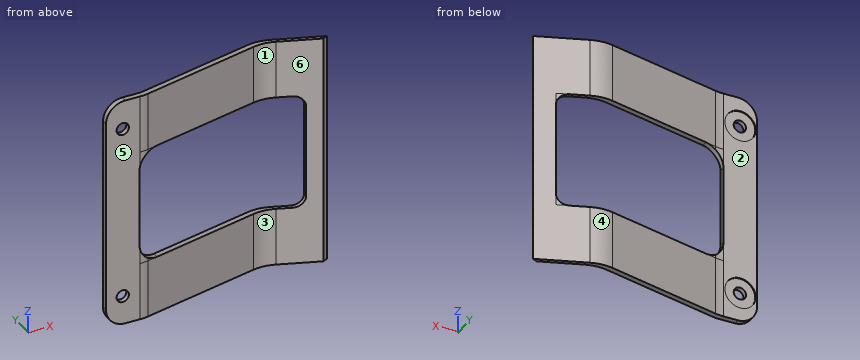
from build123d import *

# Parameters (mm, degrees)
EXTRUDE_1_DEPTH                 = 60
FILLET_1_R                      = 10
CHAMFER_1_SIZE                  = 2
CHAMFER_1_SIZE_2                = 1.558687347
CUT_EXTRUDE_1_REACH             = 86.761
SKETCH_2_R                      = 1.6
SKETCH_3_R                      = 4
CUT_EXTRUDE_2_DEPTH             = 0.2
CUT_EXTRUDE_3_REACH             = 86.761
SKETCH_4_W                      = 45.702932162
SKETCH_4_H                      = 30
CUT_EXTRUDE_3_DIRECTION_2_REACH = 86.761
FILLET_2_OUTLINE_W              = 8.702446171
FILLET_2_OUTLINE_H              = 1.5
FILLET_2_DEPTH                  = 5
FILLET_START                    = 55
FILLET_2_2_OUTLINE_W            = 8.702446171
FILLET_2_2_OUTLINE_H            = 1.5
FILLET_2_2_DEPTH                = 5
FILLET_2_3_DEPTH                = 1.3
FILLET_START_2                  = 1.3
FILLET_2_4_DEPTH                = 0.2
FILLET_START_3                  = 1.478876
FILLET_2_5_DEPTH                = 0.906082345
FILLET_START_4                  = 15
FILLET_2_6_DEPTH                = 30
FILLET_3_R                      = 3


with BuildPart() as part:
    # 草图1 → 凸台-拉伸1 (new body)
    with BuildSketch(Plane.XY):
        Polygon((0, 0), (10, 0), (45, 8), (60, 2.5), (60, 3.565103021), (44.204382552, 9.356829418), (9.830753848, 1.5), (0, 1.5), align=None)
    extrude(amount=EXTRUDE_1_DEPTH)

    # 圆角1
    fillet_1_edges = [part.edges().sort_by_distance(p)[0] for p in [
        (9.830753848, 1.5, 30),
        (44.204382552, 9.356829418, 30),
        (45, 8, 30),
        (10, 0, 30),
    ]]
    fillet(fillet_1_edges, radius=FILLET_1_R)

    # 倒角1
    # the kernel refuses this chamfer: 2, 1.558687347 mm, written as the material it takes off along each edge
    with BuildSketch(Plane(origin=(60, 2.5, -5.143365976), x_dir=(-0.9388763158866087, 0.3442546491584233, 0), z_dir=(0, 0, 1))) as chamfer_1_piece_1:
        Polygon((CHAMFER_1_SIZE, 0), (CHAMFER_1_SIZE_2 * 0.3442546492, -CHAMFER_1_SIZE_2 * 0.938876315999), (0, 0), align=None)
    extrude(amount=70.286731952, mode=Mode.SUBTRACT)

    # 草图2 → 切除-拉伸1 (cut, up to next)
    with BuildSketch(Plane(origin=(0, 1.5, 0), x_dir=(1, 0, 0), z_dir=(0, 1, 0)), mode=Mode.PRIVATE) as cut_extrude_1_sk1:
        with Locations(Location((4.351223085, -7.5, 0), (0, 0, 270))):
            Circle(SKETCH_2_R)
    cut_extrude_1_tool1 = extrude(cut_extrude_1_sk1.sketch, amount=-CUT_EXTRUDE_1_REACH, mode=Mode.PRIVATE) & part.part
    # 草图2 → 切除-拉伸1 (cut, up to next)
    with BuildSketch(Plane(origin=(0, 1.5, 0), x_dir=(1, 0, 0), z_dir=(0, 1, 0)), mode=Mode.PRIVATE) as cut_extrude_1_sk2:
        with Locations(Location((4.351223085, -52.5, 0), (0, 0, 270))):
            Circle(SKETCH_2_R)
    cut_extrude_1_tool2 = extrude(cut_extrude_1_sk2.sketch, amount=-CUT_EXTRUDE_1_REACH, mode=Mode.PRIVATE) & part.part
    add(cut_extrude_1_tool1.solids().sort_by_distance((4.351223, 1.5, 7.5))[0], mode=Mode.SUBTRACT)
    add(cut_extrude_1_tool2.solids().sort_by_distance((4.351223, 1.5, 52.5))[0], mode=Mode.SUBTRACT)

    # 草图3 → 切除-拉伸2 (cut)
    with BuildSketch(Plane(origin=(0, 1.5, 0), x_dir=(1, 0, 0), z_dir=(0, 1, 0))):
        with Locations(Location((4.351223085, -7.5, 0), (0, 0, 270))):
            Circle(SKETCH_3_R)
        with Locations(Location((4.351223085, -52.5, 0), (0, 0, 270))):
            Circle(SKETCH_3_R)
    extrude(amount=-CUT_EXTRUDE_2_DEPTH, mode=Mode.SUBTRACT)

    # 草图4 → 切除-拉伸3 (cut, up to next)
    with BuildSketch(Plane(origin=(0, 1.5, 0), x_dir=(1, 0, 0), z_dir=(0, 1, 0)), mode=Mode.PRIVATE) as cut_extrude_3_sk1:
        with Locations((31.553912252, -30)):
            Rectangle(SKETCH_4_W, SKETCH_4_H)
    cut_extrude_3_tool1 = extrude(cut_extrude_3_sk1.sketch, amount=-CUT_EXTRUDE_3_REACH, mode=Mode.PRIVATE) & part.part
    add(cut_extrude_3_tool1.solids().sort_by_distance((31.553912, 1.5, 30))[0], mode=Mode.SUBTRACT)

    # 草图4 → 切除-拉伸3 direction 2 (cut, up to next)
    with BuildSketch(Plane(origin=(0, 1.5, 0), x_dir=(1, 0, 0), z_dir=(0, 1, 0)), mode=Mode.PRIVATE) as cut_extrude_3_direction_2_sk1:
        with Locations((31.553912252, -30)):
            Rectangle(SKETCH_4_W, SKETCH_4_H)
    cut_extrude_3_direction_2_tool1 = extrude(cut_extrude_3_direction_2_sk1.sketch, amount=CUT_EXTRUDE_3_DIRECTION_2_REACH, mode=Mode.PRIVATE) & part.part
    add(cut_extrude_3_direction_2_tool1.solids().sort_by_distance((31.553912, 1.5, 30))[0], mode=Mode.SUBTRACT)

    # 圆角2: read off the stored shape, not the designer's step
    # 圆角2 outline → 圆角2 (cut)
    with BuildSketch(Plane.XY):
        with Locations((4.351223086, 0.75)):
            Rectangle(FILLET_2_OUTLINE_W, FILLET_2_OUTLINE_H)
    extrude(amount=FILLET_2_DEPTH, mode=Mode.SUBTRACT)

    # Fillet 2 2 outline → Fillet 2 2 (cut)
    with BuildSketch(Plane.XY.offset(FILLET_START)):
        with Locations((4.351223086, 0.75)):
            Rectangle(FILLET_2_2_OUTLINE_W, FILLET_2_2_OUTLINE_H)
    extrude(amount=FILLET_2_2_DEPTH, mode=Mode.SUBTRACT)

    # Fillet 2 3 outline → Fillet 2 3 (add)
    with BuildSketch(Plane(origin=(0, 0, 0), x_dir=(1, 0, 0), z_dir=(0, 1, 0))):
        with BuildLine():
            Line((5, -60), (8.702446171, -60))
            Line((8.702446171, -60), (8.702446171, -55))
            Line((8.702446171, -55), (0, -55))
            ThreePointArc((0, -55), (1.464466094, -58.535533906), (5, -60))
        make_face()
        with BuildLine():
            Line((8.702446171, -5), (8.702446171, 0))
            Line((8.702446171, 0), (5, 0))
            ThreePointArc((5, 0), (1.464466094, -1.464466094), (0, -5))
            Line((0, -5), (8.702446171, -5))
        make_face()
        with BuildLine():
            ThreePointArc((13.702446171, -45), (10.166912265, -43.535533906), (8.702446171, -40))
            Line((8.702446171, -40), (8.702446171, -45))
            Line((8.702446171, -45), (13.702446171, -45))
        make_face()
        with BuildLine():
            ThreePointArc((8.702446171, -20), (10.166912265, -16.464466094), (13.702446171, -15))
            Line((13.702446171, -15), (8.702446171, -15))
            Line((8.702446171, -15), (8.702446171, -20))
        make_face()
    extrude(amount=FILLET_2_3_DEPTH)

    # Fillet 2 4 outline → Fillet 2 4 (add)
    with BuildSketch(Plane(origin=(0, 0, 0), x_dir=(1, 0, 0), z_dir=(0, 1, 0)).offset(FILLET_START_2)):
        with BuildLine():
            Line((5, -60), (8.702446171, -60))
            Line((8.702446171, -60), (8.702446171, -55))
            Line((8.702446171, -55), (7.473722084, -55))
            ThreePointArc((7.473722084, -55), (4.351223085, -56.5), (1.228724086, -55))
            Line((1.228724086, -55), (0, -55))
            ThreePointArc((0, -55), (1.464466094, -58.535533906), (5, -60))
        make_face()
        with BuildLine():
            Line((8.702446171, -5), (8.702446171, 0))
            Line((8.702446171, 0), (5, 0))
            ThreePointArc((5, 0), (1.464466094, -1.464466094), (0, -5))
            Line((0, -5), (1.228724086, -5))
            ThreePointArc((1.228724086, -5), (4.351223085, -3.5), (7.473722084, -5))
            Line((7.473722084, -5), (8.702446171, -5))
        make_face()
        with BuildLine():
            ThreePointArc((13.702446171, -45), (10.166912265, -43.535533906), (8.702446171, -40))
            Line((8.702446171, -40), (8.702446171, -45))
            Line((8.702446171, -45), (13.702446171, -45))
        make_face()
        with BuildLine():
            ThreePointArc((8.702446171, -20), (10.166912265, -16.464466094), (13.702446171, -15))
            Line((13.702446171, -15), (8.702446171, -15))
            Line((8.702446171, -15), (8.702446171, -20))
        make_face()
    extrude(amount=FILLET_2_4_DEPTH)

    # Fillet 2 5 outline → Fillet 2 5 (add)
    with BuildSketch(Plane(origin=(0, 0, 0), x_dir=(1, 0, 0), z_dir=(0, 1, 0)).offset(FILLET_START_3)):
        with BuildLine():
            ThreePointArc((13.702446171, -45), (10.166912265, -43.535533906), (8.702446171, -40))
            Line((8.702446171, -40), (8.702446171, -45))
            Line((8.702446171, -45), (13.702446171, -45))
        make_face()
        with BuildLine():
            ThreePointArc((8.702446171, -20), (10.166912265, -16.464466094), (13.702446171, -15))
            Line((13.702446171, -15), (8.702446171, -15))
            Line((8.702446171, -15), (8.702446171, -20))
        make_face()
    extrude(amount=FILLET_2_5_DEPTH)

    # Fillet 2 6 outline → Fillet 2 6 (cut)
    with BuildSketch(Plane.XY.offset(FILLET_START_4)):
        with BuildLine():
            Line((10.930694186, 1.751414934), (13.702446193, 2.38495825))
            Line((13.702446193, 2.38495825), (8.702446171, 2.384958345))
            Line((8.702446171, 2.384958345), (8.702446171, 1.5))
            ThreePointArc((8.702446171, 1.5), (9.823639585, 1.563052515), (10.930694186, 1.751414934))
        make_face()
        with BuildLine():
            Line((8.871692322, 0), (13.702446171, 0))
            Line((13.702446171, 0), (13.702446171, 0.846273411))
            Line((13.702446171, 0.846273411), (11.099940337, 0.251414934))
            ThreePointArc((11.099940337, 0.251414934), (9.992885736, 0.063052515), (8.871692322, 0))
        make_face()
    extrude(amount=FILLET_2_6_DEPTH, mode=Mode.SUBTRACT)

    # 圆角3
    # the kernel refuses this fillet: 3 mm, written as the material it adds along each edge
    with BuildSketch(Plane(origin=(54.405378333, -2.948638722, 45), x_dir=(-1, 0, 0), z_dir=(0, 1, 0))) as fillet_3_piece_1_section:
        with BuildLine():
            CenterArc((FILLET_3_R, -FILLET_3_R), FILLET_3_R, 90, 90)
            Line((0, -FILLET_3_R), (0, 0))
            Line((0, 0), (FILLET_3_R, 0))
        make_face()
    fillet_3_piece_1 = extrude(amount=16.065103021, mode=Mode.PRIVATE)
    fillet_3_piece_1 = split(fillet_3_piece_1, bisect_by=Plane(origin=(56.829472359, 3.662526802, 45), z_dir=(0.34425464915842324, 0.9388763158866087, 0)), keep=Keep.TOP, mode=Mode.PRIVATE)
    fillet_3_piece_1 = split(fillet_3_piece_1, bisect_by=Plane(origin=(57.173727008, 4.601403118, 45), z_dir=(-0.344254649158423, -0.9388763158866088, 0)), keep=Keep.TOP, mode=Mode.PRIVATE)
    add(fillet_3_piece_1)
    with BuildSketch(Plane(origin=(54.405378333, -2.948638722, 15), x_dir=(-1, 0, 0), z_dir=(0, 1, 0))) as fillet_3_piece_2_section:
        with BuildLine():
            CenterArc((FILLET_3_R, FILLET_3_R), FILLET_3_R, 180, 90)
            Line((0, FILLET_3_R), (0, 0))
            Line((0, 0), (FILLET_3_R, 0))
        make_face()
    fillet_3_piece_2 = extrude(amount=16.065103021, mode=Mode.PRIVATE)
    fillet_3_piece_2 = split(fillet_3_piece_2, bisect_by=Plane(origin=(57.173727008, 4.601403118, 15), z_dir=(-0.344254649158423, -0.9388763158866088, 0)), keep=Keep.TOP, mode=Mode.PRIVATE)
    fillet_3_piece_2 = split(fillet_3_piece_2, bisect_by=Plane(origin=(56.829472359, 3.662526802, 15), z_dir=(0.34425464915842324, 0.9388763158866087, 0)), keep=Keep.TOP, mode=Mode.PRIVATE)
    add(fillet_3_piece_2)


solid = part.part
CAD build for the part. Positions are in the model's coordinates, mm. Face numbers are marked on the shaded views. A direction names the side the tool comes from. Coordinates: 2 decimals unless noted, no trailing zeros. Order: outer loops, then holes, each group sorted by start corner. A loop starts at its lowest first (then second) coordinate and runs counter-clockwise, first axis right, second up. Notation, with made-up numbers: (6, 16.25) -> (62, 16.25) arc R18 cw to (62, 23.25) -> close; hole circle Ø7 at (4, 87.25). An arc over 180 degrees is marked (long way). Answer in a Markdown table with one row per item.
1) Mould opens along X. For the marked faces 1, 2, 3 and 4 say: pulls with the +X half, pulls with the -X half, needs draft (parallel to the pull), parting line crosses it, or undercut.
Check values:
| item | result |
|---|---|
| face 1 | undercut |
| face 2 | needs draft |
| face 3 | undercut |
| face 4 | parting line crosses it |
2) Band-saw the part on B-B (x = 26.5). List the corners of the cut face in (y, z).
Check values:
| item | result |
|---|---|
| outline | (3.77, 0) -> (5.31, 0) -> (5.31, 15) -> (3.77, 15) -> close; (3.77, 45) -> (5.31, 45) -> (5.31, 60) -> (3.77, 60) -> close |
3) Band-saw the part on A-A (z = 52.5). List the corners of the cut face in (x, y), and give its area (3 significant figures).
Check values:
| item | result |
|---|---|
| outline | (0, 0) -> (2.75, 0) -> (2.75, 1.3) -> (0.35, 1.3) -> (0.35, 1.5) -> (0, 1.5) -> close; (5.95, 0) -> (8.87, 0) arc R10 ccw to (11.1, 0.25) -> (42.11, 7.34) arc R10 cw to (47.78, 6.98) -> (58.12, 3.19) -> (59.41, 3.78) -> (46.99, 8.34) arc R10 ccw to (41.32, 8.7) -> (10.93, 1.75) arc R10 cw to (8.7, 1.5) -> (8.35, 1.5) -> (8.35, 1.3) -> (5.95, 1.3) -> close |
| area | 77.6 mm2 |
4) Band-saw the part on C-C (z = 23). List the corners of the cut face in (x, y), and give its area (3 significant figures).
Check values:
| item | result |
|---|---|
| outline | (0, 0) -> (8.7, 0) -> (8.7, 1.5) -> (0, 1.5) -> close; (54.41, 4.55) -> (58.12, 3.19) -> (59.41, 3.78) -> (54.41, 5.62) -> close |
| area | 17.7 mm2 |
5) Drill centre lines: line 1 (Y direction, x = 48.5, z = 13); line 2 (Y direction, x = 19.5, z = 54). Where is each one in solid material? Low to high.
Check values:
| item | result |
|---|---|
| line 1 | 6.72 to 7.78 |
| line 2 | 2.17 to 3.71 |
6) Flat gauge pins, fed straight in: P1, Ø2, axis at x = 20, y = 6, coming from the +Z side; P2, Ø10, axis at x = 42, z = 13.5, coming from the -Y side; P3, Ø9.5, axis at x = 5, z = 33.5, coming from the +Y side; P4, Ø4, axis at x = 4.35, z = 7.5, coming from the +Y side. Where does each tip first touch, or does it go through?
Check values:
| item | result |
|---|---|
| P1 | through |
| P2 | y = 6.17 |
| P3 | y = 1.5 |
| P4 | y = 1.3 |
7) Which spindle directions (+Z, -Z, +X, -X, +Y, -Y) get a long thin tool onto all of the face, cutting with end or side? Do the marked faces 5 and 6. Say none if no direction does.
Check values:
| item | result |
|---|---|
| face 5 | +Z, -Z, +X, -X, -Y |
| face 6 | +Z, -Z, -Y |
